```python
from build123d import *

# Parameters (mm, degrees)
BOSS_EXTRUDE1_DEPTH = 3.18
SKETCH2_W           = 2.8
SKETCH2_H           = 9
SKETCH2_H_2         = 6
CUT_EXTRUDE1_DEPTH  = 153.716608134


with BuildPart() as part:
    # Sketch1 → Boss-Extrude1 (new body)
    with BuildSketch(Plane.XY):
        Polygon((-10.795, 0), (-10.795, -3), (-17.915, -3), (-17.915, 0), (-28.5, 0), (-28.5, 150), (0, 150), (0, 0), align=None)
    extrude(amount=BOSS_EXTRUDE1_DEPTH)

    # Sketch2 → Cut-Extrude1 (cut, through all)
    with BuildSketch(Plane.XY.offset(3.18)):
        with Locations((-27.1, 13.5)):
            Rectangle(SKETCH2_W, SKETCH2_H)
        with Locations((-27.1, 31.5)):
            Rectangle(SKETCH2_W, SKETCH2_H)
        with Locations((-27.1, 49.5)):
            Rectangle(SKETCH2_W, SKETCH2_H)
        with Locations((-27.1, 67.5)):
            Rectangle(SKETCH2_W, SKETCH2_H)
        with Locations((-27.1, 85.5)):
            Rectangle(SKETCH2_W, SKETCH2_H)
        with Locations((-27.1, 103.5)):
            Rectangle(SKETCH2_W, SKETCH2_H)
        with Locations((-27.1, 121.5)):
            Rectangle(SKETCH2_W, SKETCH2_H)
        with Locations((-27.1, 139.5)):
            Rectangle(SKETCH2_W, SKETCH2_H)
        with Locations((-1.4, 4.5)):
            Rectangle(SKETCH2_W, SKETCH2_H)
        with Locations((-1.4, 22.5)):
            Rectangle(SKETCH2_W, SKETCH2_H)
        with Locations((-1.4, 40.5)):
            Rectangle(SKETCH2_W, SKETCH2_H)
        with Locations((-1.4, 58.5)):
            Rectangle(SKETCH2_W, SKETCH2_H)
        with Locations((-1.4, 76.5)):
            Rectangle(SKETCH2_W, SKETCH2_H)
        with Locations((-1.4, 94.5)):
            Rectangle(SKETCH2_W, SKETCH2_H)
        with Locations((-1.4, 112.5)):
            Rectangle(SKETCH2_W, SKETCH2_H)
        with Locations((-1.4, 130.5)):
            Rectangle(SKETCH2_W, SKETCH2_H)
        with Locations((-1.4, 147)):
            Rectangle(SKETCH2_W, SKETCH2_H_2)
    extrude(amount=-CUT_EXTRUDE1_DEPTH, mode=Mode.SUBTRACT)


solid = part.part
```
Check sheet for the modelled part. Datum: model origin and axes. Units: mm. A direction names the side the tool comes from. Round coordinates to 2 decimals unless told otherwise and drop trailing zeros. Loops run counter-clockwise (first coordinate to the right, second up) from the corner with the lowest first, then second, coordinate; pieces in that order, holes last. Notation, with made-up numbers: (30, 40.25) - (43, 40.25) arc R7 ccw to (43, 50.25) - close; hole circle Ø6 at (50.25, 84.25). An arc over 180 degrees is marked (long way). Write item = value, one per line. Start each with the question number.
Q1. Access from +Z, -Z, +X, -X, +Y, -Y to the whole of each face (thin tool, end or side, straight path). Record for faces 1 (the face through (-2.8, 58, 2)), 2 (the face through (-7, 0, 2)), 3 (the face through (-25.7, 121, 2)).
Q2. Release check for a two-part mould opening along Y. For faces 4 (the face through (-25.7, 85, 2)), 5 (the face through (-23, 0, 2)), 6 (the face through (-28.5, 147, 2)) record: pulls with the +Y half, pulls with the -Y half, needs draft (parallel to the pull), parting line crosses it, or undercut.
Q3. Thickness scan on L1, parallel to Y at x = -9.25, z = 2.35; L2, parallel to X at y = 140.5, z = 0.35; L3, parallel to X at y = 111.5, z = 1.6. Record the ranges inside material, lowest first.
Q4. Depth check by flat-ended pin: P1, Ø1, axis at y = 127, z = 1.5, coming from the +X side; P2, Ø1.5, axis at x = -6, z = 2, coming from the -Y side; P3, Ø0.8, axis at x = -0.5, z = 1, coming from the +Y side. Enter the tip coordinate at first touch or a pass-through.
Q5. Section check A-A (y = 32.5). Record the boundary of the cut face in (x, z).
Q6. Section check B-B (x = -23.75). Record the boundary of the cut face in (y, z).
Derived:
q1.face_1 = +Z, -Z, +X
q1.face_2 = +Z, -Z, +X, -Y
q1.face_3 = +Z, -Z, -X
q2.face_4 = undercut
q2.face_5 = pulls with the -Y half
q2.face_6 = needs draft
q3.L1 = 0 to 150
q3.L2 = -25.7 to 0
q3.L3 = -28.5 to -2.8
q4.P1 = -2.8
q4.P2 = 0
q4.P3 = 144
q5.outline = (-25.7, 0) - (0, 0) - (0, 3.18) - (-25.7, 3.18) - close
q6.outline = (0, 0) - (150, 0) - (150, 3.18) - (0, 3.18) - close
